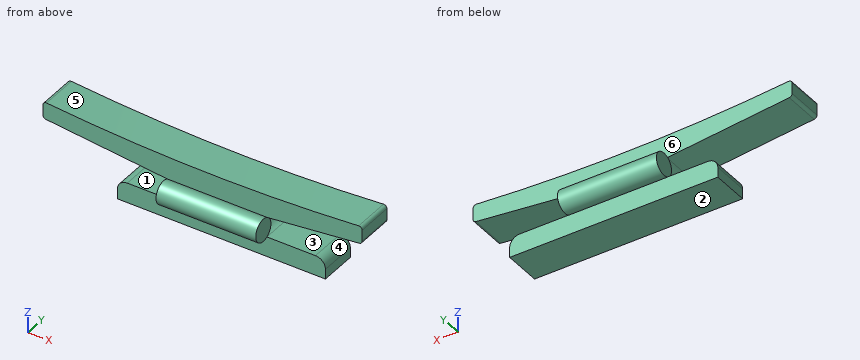
```python
from build123d import *

# Parameters (mm, degrees)
F1_DEPTH = 23.8125
F2_R     = 7.251035
F3_DEPTH = 31.496
F4_DEPTH = 31.75


with BuildPart() as f1:
    # F0 (on Front) → F1 (new body)
    with BuildSketch(Plane.XZ):
        with BuildLine():
            Line((-63.5, -4.98963), (-63.5, -11.33963))
            Line((-63.5, -11.33963), (0, -11.33963))
            Line((0, -11.33963), (69.038319, -11.33963))
            Line((69.038319, -11.33963), (69.038319, -4.98963))
            ThreePointArc((69.038319, -4.98963), (67.178447, -0.499502), (62.688319, 1.36037))
            Line((62.688319, 1.36037), (31.75, 1.36037))
            ThreePointArc((31.75, 1.36037), (25.409083, 7.37086), (31.071951, 14.024066))
            Line((31.071951, 14.024066), (90.570115, 20.413778))
            ThreePointArc((90.570115, 20.413778), (91.864747, 21.076197), (92.385139, 22.434161))
            Line((92.385139, 22.434161), (92.385139, 29.566896))
            ThreePointArc((92.385139, 29.566896), (91.732126, 31.05935), (90.192796, 31.59256))
            ThreePointArc((90.192796, 31.59256), (-9.233486, 28.065795), (-108.589812, 33.198436))
            ThreePointArc((-108.589812, 33.198436), (-110.149746, 32.679172), (-110.814861, 31.175627))
            Line((-110.814861, 31.175627), (-110.814861, 24.413392))
            ThreePointArc((-110.814861, 24.413392), (-110.294469, 23.055428), (-108.999837, 22.393009))
            Line((-108.999837, 22.393009), (-31.071951, 14.024066))
            ThreePointArc((-31.071951, 14.024066), (-25.409083, 7.37086), (-31.75, 1.36037))
            Line((-31.75, 1.36037), (-57.15, 1.36037))
            ThreePointArc((-57.15, 1.36037), (-61.640128, -0.499502), (-63.5, -4.98963))
        make_face()
    extrude(amount=F1_DEPTH)

    # F2 (on Right) → F3 (join, symmetric)
    with BuildSketch(Plane.YZ):
        with Locations((3.39075, 7.690888)):
            Circle(F2_R)
    extrude(amount=F3_DEPTH, both=True)

    # F2 (on Right) → F4 (join, symmetric)
    with BuildSketch(Plane.YZ):
        with Locations((-27.20325, 7.690888)):
            Circle(F2_R)
    extrude(amount=F4_DEPTH, both=True)


solid = f1.part
```
Source: CAD feature listing. Evaluate the final solid. Frame: model axes, mm. Face numbers are marked on the shaded views. A direction names the side the tool comes from. Give positions to 0.01 mm unless a question says otherwise; leave off trailing zeros. Loops run counter-clockwise (first coordinate to the right, second up) from the corner with the lowest first, then second, coordinate; pieces in that order, holes last. Notation, with made-up numbers: (1.5, -14) -> (37.5, -14) arc R36 ccw to (37.5, 20) -> close; hole circle Ø9 at (-7.75, 71). An arc over 180 degrees is marked (long way). Put each result on its own line as item: value. Start each with the question number.
1) Cut plane C-C (y = -10). Return loops of the section in (x, z).
2) Draft query along Z for the marked faces 4, 5 and 6. Return one class per face: released by +Z, released by -Z, zero draft, split by the parting line, or undercut.
3) Reachability of the marked faces 1, 2 and 3 from +Z, -Z, +X, -X, +Y, -Y: full face, straight path, thin tool, end or side. Return the list, or none.
4) Cut plane A-A (z = 5). Return loops of the section in (x, y).
5) Cut plane D-D (y = -27.5). Return loops of the section in (x, z), then the cut area to 3 significant figures.
6) Cut plane B-B (x = -5.5). Return loops of the section in (y, z), then the cut area to 3 significant figures.
7) Material intervals for probe 1 along Y at (x, z) = (34, 25.5); probe 2 along Y at (x, z) = (7, 7); probe 3 along X at (y, z) = (8.5, 7), sorted ascending.
8) Contact query for flat-ended pins moving along their axis: P1, Ø14, axis at x = 19.5, z = -2, coming from the +Y side; P2, Ø11.5, axis at y = -28, z = 8, coming from the +X side; P3, Ø3, axis at y = -16.5, z = -8, coming from the -X side. Output: stop coordinate, or through.
Results are:
1. outline: (-110.81, 24.41) arc R2.03 ccw to (-109, 22.39) -> (-31.07, 14.02) arc R6.35 cw to (-31.75, 1.36) -> (-57.15, 1.36) arc R6.35 ccw to (-63.5, -4.99) -> (-63.5, -11.34) -> (69.04, -11.34) -> (69.04, -4.99) arc R6.35 ccw to (62.69, 1.36) -> (31.75, 1.36) arc R6.35 cw to (31.07, 14.02) -> (90.57, 20.41) arc R2.03 ccw to (92.39, 22.43) -> (92.39, 29.57) arc R2.03 ccw to (90.19, 31.59) arc R1143 cw to (-108.59, 33.2) arc R2.03 ccw to (-110.81, 31.18) -> close
2. face 4: undercut
2. face 5: released by +Z
2. face 6: zero draft
3. face 1: -X, +Y, -Y
3. face 2: -Z, +X, -X, +Y, -Y
3. face 3: +X, +Y, -Y
4. outline: (-31.75, -33.94) -> (31.75, -33.94) -> (31.75, -20.47) -> (26.01, -20.47) -> (26.01, -3.34) -> (31.5, -3.34) -> (31.5, 10.12) -> (-31.5, 10.12) -> (-31.5, -3.34) -> (-26.01, -3.34) -> (-26.01, -20.47) -> (-31.75, -20.47) -> close
5. outline: (-31.75, 0.45) -> (31.75, 0.45) -> (31.75, 14.94) -> (-31.75, 14.94) -> close
5. area: 920 mm2
6. outline: (-23.81, -11.34) -> (0, -11.34) -> (0, 1.28) arc R7.25 ccw (long way) to (0, 14.1) -> (0, 28.04) -> (-23.81, 28.04) -> (-23.81, 14.1) arc R7.25 ccw (long way) to (-23.81, 1.28) -> close
6. area: 1,200 mm2
7. probe 1: y = -23.81 to 0
7. probe 2: y = -34.42 to 10.61
7. probe 3: x = -31.5 to 31.5
8. P1: stops at y = 10.12
8. P2: stops at x = 31.75
8. P3: stops at x = -63.5
